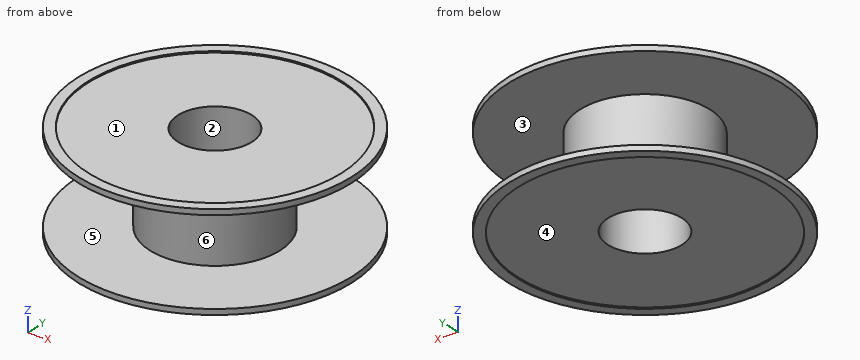
Autodesk Inventor part; units mm, degrees
ref_plane "Work Plane1" through (0, 0, -31) normal (0, 0, -1) x (-1, 0, 0)
ref_plane "YZ Plane" through (0, 0, 0) normal (1, 0, 0) x (0, 1, 0)
ref_plane "XZ Plane" through (0, 0, 0) normal (0, 1, 0) x (-1, 0, 0)
sketch "Sketch11" plane through (0, 0, 0) normal (0, 0, 1) x (1, 0, 0)
  circle A0 centre (0, 0) radius 100
  dimension "d39" = 200
extrude "Extrusion10" add sketch "Sketch11" along normal blind 4
sketch "Sketch12" plane through (0, 0, 4) normal (0, 0, 1) x (1, 0, 0)
  circle A0 centre (0, 0) radius 100
  circle A1 centre (0, 0) radius 92.5
  dimension "d42" = 185
extrude "Extrusion11" cut sketch "Sketch12" against normal blind 1 contours A1
ref_plane "Work Plane1" through (0, 0, -31) normal (0, 0, -1) x (-1, 0, 0)
mirror "Mirror1" about plane through (0, 0, -31) normal (0, 0, -1)
sketch "Sketch14" plane through (0, 0, -62) normal (0, 0, 1) x (1, 0, 0)
  circle A0 centre (0, 0) radius 100
  circle A1 centre (0, 0) radius 47.5
  dimension "d46" = 95
extrude "Extrusion12" add sketch "Sketch14" along normal up to next contours A1
sketch "Sketch15" plane through (0, 0, -65) normal (0, 0, -1) x (-1, 0, 0)
  circle A0 centre (0, 0) radius 92.5
  circle A1 centre (0, 0) radius 27
  dimension "d50" = 54
extrude "Extrusion13" cut sketch "Sketch15" against normal up to surface (68 mm away) contours A1
properties part number "SpoolFilamentToyBuilder" material "ABS Plastic"
Geometry check sheet. Reference: the model listing, model coordinates, mm. Face numbers are marked on the shaded views. A direction names the side the tool comes from. Round coordinates to 2 decimals unless told otherwise and drop trailing zeros. Order: outer loops, then holes, each group sorted by start corner. A loop starts at its lowest first (then second) coordinate and runs counter-clockwise, first axis right, second up. Notation, with made-up numbers: (52.25, 9) -> (72.25, 9) arc R20 cw to (72.25, 13) -> close; hole circle Ø9 at (3.5, -28). An arc over 180 degrees is marked (long way). Use one line per item in the form item = value.
1. Set-up check for the marked faces 1, 2 and 3: record each of +Z, -Z, +X, -X, +Y, -Y from which the full face is reachable in a straight line by a thin tool's end or side.
Working result:
face_1 = +Z
face_2 = +Z, -Z
face_3 = none
2. Cross-section at A-A, the plane y = 0. Enter the section's corners in (x, z), plus the area to 3 significant figures.
Working result:
outline = (-100, -66) -> (-92.5, -66) -> (-92.5, -65) -> (-27, -65) -> (-27, 3) -> (-92.5, 3) -> (-92.5, 4) -> (-100, 4) -> (-100, 0) -> (-47.5, 0) -> (-47.5, -62) -> (-100, -62) -> close; (27, -65) -> (92.5, -65) -> (92.5, -66) -> (100, -66) -> (100, -62) -> (47.5, -62) -> (47.5, 0) -> (100, 0) -> (100, 4) -> (92.5, 4) -> (92.5, 3) -> (27, 3) -> close
area = 3,450 mm^2
3. Mould release check, pull along Y, two halves, no side actions. Record for the marked faces 4, 5 and 6: pulls with the +Y half, pulls with the -Y half, needs draft (parallel to the pull), parting line crosses it, or undercut.
Working result:
face_4 = undercut
face_5 = needs draft
face_6 = parting line crosses it
4. Scan lines: line 1 along Z through (x, y) = (-10, -51); line 2 along Y through (x, z) = (0, 3.6); line 3 along Z through (x, y) = (-76, -62). Record each from-to range of solid material in increasing order. Write a range as from..to.
Working result:
line_1 = -65..-62, 0..3
line_2 = -100..-92.5, 92.5..100
line_3 = -66..-62, 0..4
5. Cross-section at C-C, the plane z = -9. Enter the section's corners in (x, y).
Working result:
outline = circle Ø95 at (0, 0); hole circle Ø54 at (0, 0)
6. Go/stop test with flat-tipped pins: pin 1 (4 mm diameter, centred on x = 64.5, y = 3, fed in from +Z); pin 2 (2 mm diameter, centred on x = 34, z = -57.5, fed in from +Y); pin 3 (5 mm diameter, centred on x = 9, z = -8, fed in from -Y). Record where each tip stops, or that it passes through.
Working result:
pin_1 = 3
pin_2 = 34.17
pin_3 = -47.05
7. Cross-section at D-D, the plane y = 59.5. Enter the section's corners in (x, z), plus the area to 3 significant figures.
Working result:
outline = (-80.37, -66) -> (-70.82, -66) -> (-70.82, -65) -> (70.82, -65) -> (70.82, -66) -> (80.37, -66) -> (80.37, -62) -> (-80.37, -62) -> close; (-80.37, 0) -> (80.37, 0) -> (80.37, 4) -> (70.82, 4) -> (70.82, 3) -> (-70.82, 3) -> (-70.82, 4) -> (-80.37, 4) -> close
area = 1,000 mm^2
